Autodesk Fusion 360 part; units mm, degrees
sketch "Sketch1" plane through (0, 0, 0) normal (0, 0, 1) x (1, 0, 0)
  circle A0 centre (0, 0) radius 3.275
  circle A1 centre (210, 0) radius 3.275
  circle A2 centre (0, 0) radius 15
  circle A3 centre (210, 0) radius 15
  line L0 (0, 15) -> (210, 15)
  line L1 (0, -15) -> (210, -15)
  circle A4 centre (0, 0) radius 20 construction
  circle A5 centre (210, 0) radius 20 construction
  circle A6 centre (75, 80.4674) radius 3.275
  circle A7 centre (135, 80.4674) radius 3.275
  circle A8 centre (75, 80.4674) radius 15
  circle A9 centre (135, 80.4674) radius 15
  line L2 (-10.9728, 10.2273) -> (64.0272, 90.6947)
  line L3 (75, 95.4674) -> (135, 95.4674)
  line L4 (145.9728, 90.6947) -> (220.9728, 10.2273)
  circle A10 centre (34.0909, 36.5761) radius 30 construction
  circle A11 centre (75, 80.4674) radius 30 construction
  circle A12 centre (175.9091, 36.5761) radius 30 construction
  circle A13 centre (135, 80.4674) radius 30 construction
  line L5 (0, 0) -> (75, 80.4674) construction
  circle A14 centre (34.0909, 36.5761) radius 3.275
  circle A15 centre (175.9091, 36.5761) radius 3.275
  line L6 (10.9728, -10.2273) -> (85.9728, 70.2401)
  line L7 (199.0272, -10.2273) -> (124.0272, 70.2401)
  line L8 (85.9728, 70.2401) -> (124.0272, 70.2401)
  dimension "d2" = 6.55
  dimension "d3" = 6.55
  dimension "d4" = 210
  dimension "d6" = 30
  dimension "d7" = 30
  dimension "d10" = 40
  dimension "d11" = 40
  dimension "d14" = 6.55
  dimension "d15" = 6.55
  dimension "d16" = 30
  dimension "d17" = 30
  dimension "d20" = 60
  dimension "d21" = 60
  dimension "d22" = 60
  dimension "d23" = 60
  dimension "d24" = 6.55
  dimension "d25" = 6.55
extrude "Extrude1" add sketch "Sketch1" along normal blind 5 contours A2 | A2 L0 L6 | A2 L0 A8 L2 L6 | A8 | A3 L0 A9 L4 L7 | A3 L0 L7 | A8 A9 L3 L8 | A3 | A9
equation "SlipGearNominal = 209.5 mm"
equation "d4 = SlipGearNominal + SlipGearOffset"
equation "SlipGearOffset = 0.5 mm"
CAD build for the part. Positions are in the model's coordinates, mm. A direction names the side the tool comes from. Round coordinates to 2 decimals unless told otherwise and drop trailing zeros. Write each loop counter-clockwise with the first axis right and the second up, starting at its lowest first coordinate (ties: lowest second). Pieces come first, ordered by that corner, then holes. Notation, with made-up numbers: (36, 30) -> (69, 30) arc R9 cw to (69, 42) -> close; hole circle Ø1 at (-34.75, 40). An arc over 180 degrees is marked (long way). Answer as a JSON object with one key per item and string values.
(1) Band-saw the part on A-A, the plane x = 210. List the corners of the cut face in (y, z) (3 decimals), then the cut area to 3 significant figures.
Reported:
{"outline": "(-15, 0) -> (-3.275, 0) -> (-3.275, 5) -> (-15, 5) -> close; (3.275, 0) -> (22, 0) -> (22, 5) -> (3.275, 5) -> close", "area": "152 mm^2"}
(2) Two-plate mould, pull along X, no slides. Class faces 3 (the face through (172.637, 36.432, 2.465)), 4 (the face through (26.002, 49.898, 2.465)), 5 (the face through (104, 77, 5)): +X half, -X half, draft (parallel to the pull), parting line (faces both ways), or undercut.
Reported:
{"face 3": "undercut", "face 4": "-X half", "face 5": "draft"}
(3) Band-saw the part on D-D, the plane x = 96. List the corners of the cut face in (y, z), then the cut area to 3 significant figures.
Reported:
{"outline": "(70.24, 0) -> (95.47, 0) -> (95.47, 5) -> (70.24, 5) -> close", "area": "126 mm^2"}
(4) Band-saw the part on B-B, the plane y = 8. List the corners of the cut face in (x, z), then the cut area to 3 significant figures.
Reported:
{"outline": "(-12.69, 0) -> (27.96, 0) -> (27.96, 5) -> (-12.69, 5) -> close; (182.04, 0) -> (222.69, 0) -> (222.69, 5) -> (182.04, 5) -> close", "area": "407 mm^2"}
(5) Pin check, flat tips, straight feed: P1, Ø1.5, axis at y = 2, z = 3.5, coming from the -X side; P2, Ø10.5, axis at x = 210, y = 0, coming from the -Z side; P3, Ø1.5, axis at y = 31.5, z = 1.5, coming from the -X side; P4, Ø1, axis at y = 59, z = 3.5, coming from the -X side. Stop position of each tip, or through.
Reported:
{"P1": "stops at x = -14.95", "P2": "stops at z = 0", "P3": "stops at x = 8.16", "P4": "stops at x = 34.02"}
(6) Which spindle directions (+Z, -Z, +X, -X, +Y, -Y) get a long thin tool onto all of the face, cutting with end or side? Do faces 1 (the face through (182.95, 51.02, 2.46)), 2 (the face through (162.052, 29.443, 2.465)). Say none if no direction does.
Reported:
{"face 1": "+Z, -Z, +X, +Y", "face 2": "+Z, -Z, -Y"}
(7) Probe probe 1 along X at (y, z) = (38.5, 1.55); probe 2 along Y at (x, z) = (75, 1.4); probe 3 along X at (y, z) = (41.5, 2.35). List the from-to ranges inside material, lowest first. Write a range as [from, to].
Reported:
{"probe 1": "x = [15.38, 31.44], [36.74, 56.39], [153.61, 173.26], [178.56, 194.62]", "probe 2": "y = [58.47, 77.19], [83.74, 95.47]", "probe 3": "x = [18.18, 59.19], [150.81, 191.82]"}
(8) Band-saw the part on C-C, the plane z = 0.9. List the corners of the cut face in (x, y) (3 decimals), then the cut area to 3 significant figures.
Reported:
{"outline": "(-10.973, 10.227) arc R15 ccw to (10.973, -10.227) -> (85.973, 70.24) -> (124.027, 70.24) -> (199.027, -10.227) arc R15 ccw to (220.973, 10.227) -> (145.973, 90.695) arc R15 ccw to (135, 95.467) -> (75, 95.467) arc R15 ccw to (64.027, 90.695) -> close; hole circle Ø6.55 at (0, 0); hole circle Ø6.55 at (34.091, 36.576); hole circle Ø6.55 at (75, 80.467); hole circle Ø6.55 at (135, 80.467); hole circle Ø6.55 at (175.909, 36.576); hole circle Ø6.55 at (210, 0)", "area": "8,690 mm^2"}
